Model file for the job. Use its own axes, mm. Face numbers are marked on the shaded views. A direction names the side the tool comes from. Give positions to 0.01 mm unless a question says otherwise; leave off trailing zeros. Order: outer loops, then holes, each group sorted by start corner. A loop starts at its lowest first (then second) coordinate and runs counter-clockwise, first axis right, second up. Notation, with made-up numbers: (31.5, 75.5) - (47.5, 75.5) arc R26 cw to (47.5, 99.5) - close; hole circle Ø7 at (-4, -3). An arc over 180 degrees is marked (long way). Use CSV: the item, a comma, the result in double quotes. Start each with the question number.
(1) Probe L1, parallel to Y at x = 0, z = 5.5; L2, parallel to Y at x = 0, z = 1.75; L3, parallel to Z at x = -10.5, y = 9.5. List the from-to ranges inside material, lowest first.
(2) Drop flat-ended pins along their axis: pin 1 Ø3 at (x, y) = (16.5, -9.5) entering from +Z; pin 2 Ø22.5 at (x, y) = (2, 6) entering from +Z; pin 3 Ø1 at (x, z) = (15.5, 2) entering from +Y; pin 4 Ø1 at (x, z) = (2, 5.5) entering from -Y. Give the stop position or say it passes through.
(3) Band-saw the part on D-D, the plane y = 18. Give the cut face in (x, z).
(4) Band-saw the part on C-C, the plane z = 3. Give the cut face in (x, y), then the cut area to 3 significant figures.
(5) Tool access for the marked faces 1 and 2: list every direction of +Z, -Z, +X, -X, +Y, -Y with a clear straight run to the whole face (end or side of a thin tool).
(6) Band-saw the part on A-A, the plane x = 0. Give the cut face in (y, z).
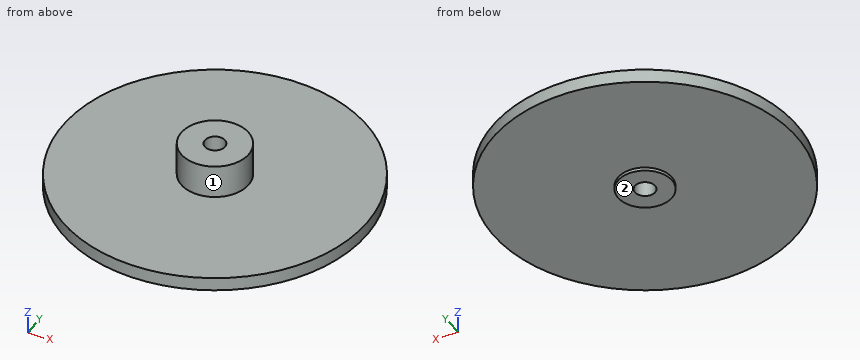
Autodesk Inventor part; units mm, degrees
ref_plane "YZ Plane" through (0, 0, 0) normal (1, 0, 0) x (0, 1, 0)
ref_plane "XZ Plane" through (0, 0, 0) normal (0, 1, 0) x (-1, 0, 0)
ref_plane "XY Plane" through (0, 0, 0) normal (0, 0, 1) x (1, 0, 0)
sketch "スケッチ1" plane through (0, 0, 0) normal (0, 0, 1) x (1, 0, 0)
  circle A0 centre (0, 0) radius 22.5
  dimension "d0" = 45
extrude "押し出し1" add sketch "スケッチ1" along normal blind 2
sketch "スケッチ2" plane through (0, 0, 2) normal (0, 0, 1) x (1, 0, 0)
  circle A0 centre (0, 0) radius 5
  dimension "d3" = 10
extrude "押し出し2" add sketch "スケッチ2" along normal blind 5
sketch "スケッチ3" plane through (0, 0, 0) normal (0, 0, -1) x (-1, 0, 0)
  circle A0 centre (0, 0) radius 4
  dimension "d6" = 8
extrude "押し出し3" add sketch "スケッチ3" along normal blind 0.5
sketch "スケッチ4" plane through (0, 0, 7) normal (0, 0, 1) x (1, 0, 0)
  circle A0 centre (0, 0) radius 1.5
  dimension "d9" = 3
extrude "押し出し4" cut sketch "スケッチ4" against normal blind 12
properties part number "Gear2_S50B 90B+0203" material "真鍮"
Answer block:
1,L1,"y = -5 to -1.5, 1.5 to 5"
1,L2,"y = -22.5 to -1.5, 1.5 to 22.5"
1,L3,"z = 0 to 2"
2,pin 1,"stops at z = 2"
2,pin 2,"stops at z = 7"
2,pin 3,"stops at y = 16.77"
2,pin 4,"stops at y = -4.77"
3,outline,"(-13.5, 0) - (13.5, 0) - (13.5, 2) - (-13.5, 2) - close"
4,outline,"circle Ø10 at (0, 0); hole circle Ø3 at (0, 0)"
4,area,"71.5 mm2"
5,face 1,"+Z"
5,face 2,"-Z, +X, -X, +Y, -Y"
6,outline,"(-22.5, 0) - (-4, 0) - (-4, -0.5) - (-1.5, -0.5) - (-1.5, 7) - (-5, 7) - (-5, 2) - (-22.5, 2) - close; (1.5, -0.5) - (4, -0.5) - (4, 0) - (22.5, 0) - (22.5, 2) - (5, 2) - (5, 7) - (1.5, 7) - close"
